Drawing for the job (mm, zero at the part's lowest x, y, z). Coordinates: 2 decimals unless noted, no trailing zeros. Write each loop counter-clockwise with the first axis right and the second up, starting at its lowest first coordinate (ties: lowest second). Pieces come first, ordered by that corner, then holes. Notation, with made-up numbers: (82, 62) - (130, 62) arc R35 cw to (130, 97) - close; hole circle Ø10 at (74.5, 18.25). An arc over 180 degrees is marked (long way). Write each question's results on one line, items separated by ' | '.
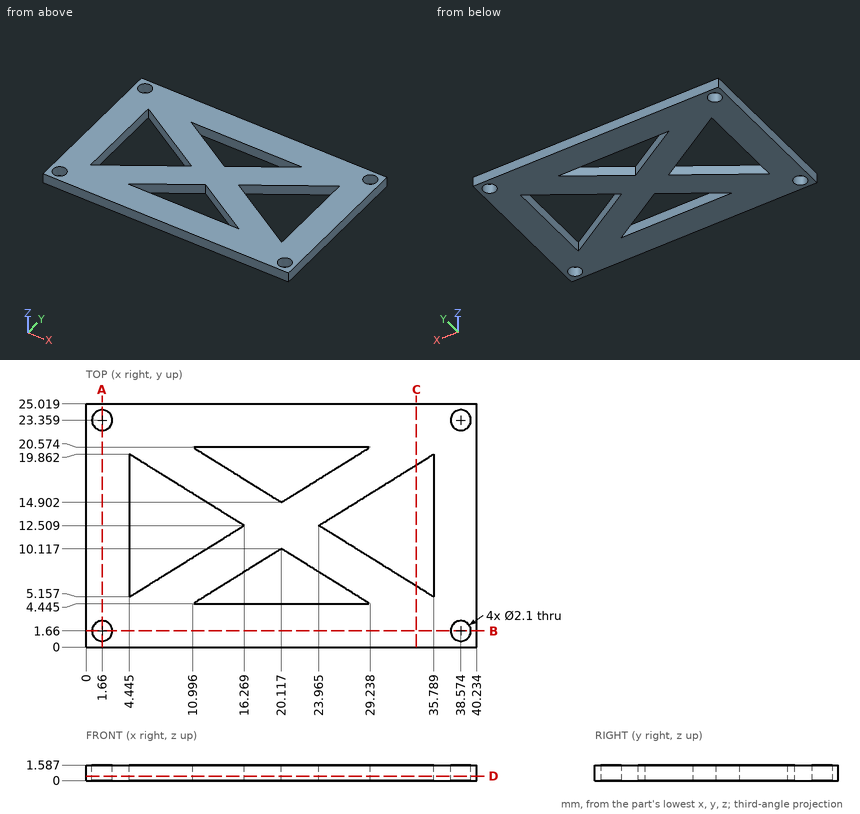
(1) Wall check: line 1 (Y direction, x = 1.66, z = 0.5); line 2 (Y direction, x = 27.5, z = 1.2) (1 decimal); line 3 (Y direction, x = 25, z = 1.4) (1 decimal). Give the ranges that are in metal, low to high. Write a range as from..to.
Return value:
line 1: y = 0..0.61, 2.71..22.31, 24.41..25.02 | line 2: y = 0..4.4, 5.5..10.3, 14.7..19.5, 20.6..25 | line 3: y = 0..4.4, 7.1..11.9, 13.2..17.9, 20.6..25
(2) Saw through at D-D on z = 0.45. Count the separate pieces of the cut face and the enclosed holes in it.
Return value:
separate pieces: 1 | enclosed holes: 8
(3) Saw through at C-C on x = 34. Write the cut outline in (y, z).
Return value:
outline: (0, 0) - (6.27, 0) - (6.27, 1.59) - (0, 1.59) - close; (18.75, 0) - (25.02, 0) - (25.02, 1.59) - (18.75, 1.59) - close
(4) Saw through at A-A on x = 1.66. Write the cut outline in (y, z).
Return value:
outline: (0, 0) - (0.61, 0) - (0.61, 1.59) - (0, 1.59) - close; (2.71, 0) - (22.31, 0) - (22.31, 1.59) - (2.71, 1.59) - close; (24.41, 0) - (25.02, 0) - (25.02, 1.59) - (24.41, 1.59) - close
(5) Saw through at B-B on y = 1.66. Write the cut outline in (x, z).
Return value:
outline: (0, 0) - (0.61, 0) - (0.61, 1.59) - (0, 1.59) - close; (2.71, 0) - (37.52, 0) - (37.52, 1.59) - (2.71, 1.59) - close; (39.62, 0) - (40.23, 0) - (40.23, 1.59) - (39.62, 1.59) - close
